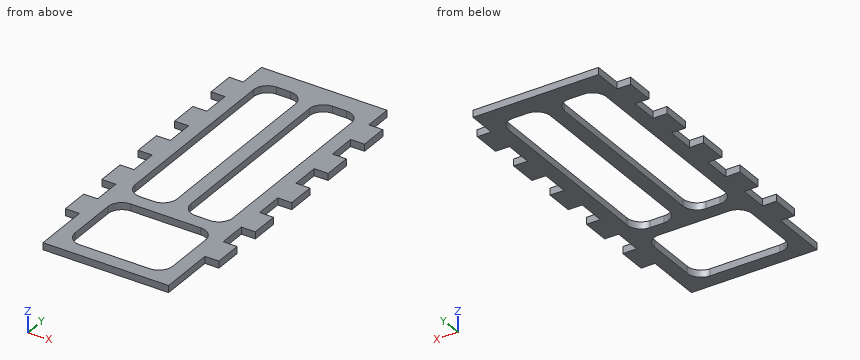
from build123d import *

# Parameters (mm, degrees)
SKETCH1_W           = 57.15
SKETCH1_H           = 152.4
BOSS_EXTRUDE1_DEPTH = 3.175
SKETCH2_W           = 6.35
SKETCH2_H           = 12.7
BOSS_EXTRUDE2_DEPTH = 3.175
LPATTERN1_COUNT     = 5
LPATTERN1_PITCH     = 25.4
SKETCH3_W           = 44.45
SKETCH3_H           = 35.56
CUT_EXTRUDE1_DEPTH  = 3.175
SKETCH4_W           = 19.05
SKETCH4_H           = 95.25
CUT_EXTRUDE2_DEPTH  = 3.175
FILLET1_R           = 6.35


with BuildPart() as part:
    # Sketch1 → Boss-Extrude1 (new body)
    with BuildSketch(Plane.XY):
        with Locations((28.575, 76.2)):
            Rectangle(SKETCH1_W, SKETCH1_H)
    extrude(amount=BOSS_EXTRUDE1_DEPTH)

    # Sketch2 → Boss-Extrude2 (add)
    with BuildSketch(Plane.XY.offset(3.175)):
        with Locations((-3.175, 133.35)):
            Rectangle(SKETCH2_W, SKETCH2_H)
        with Locations((60.325, 133.35)):
            Rectangle(SKETCH2_W, SKETCH2_H)
    boss_extrude2 = extrude(amount=-BOSS_EXTRUDE2_DEPTH)

    # LPattern1: Boss-Extrude2 ×5
    with Locations(*[(0, -i * LPATTERN1_PITCH, 0) for i in range(1, LPATTERN1_COUNT)]):
        add(boss_extrude2)

    # Sketch3 → Cut-Extrude1 (cut)
    with BuildSketch(Plane.XY.offset(3.175)):
        with Locations((28.575, 24.13)):
            Rectangle(SKETCH3_W, SKETCH3_H)
    extrude(amount=-CUT_EXTRUDE1_DEPTH, mode=Mode.SUBTRACT)

    # Sketch4 → Cut-Extrude2 (cut)
    with BuildSketch(Plane.XY.offset(3.175)):
        with Locations((15.875, 95.885)):
            Rectangle(SKETCH4_W, SKETCH4_H)
        with Locations((41.275, 95.885)):
            Rectangle(SKETCH4_W, SKETCH4_H)
    extrude(amount=-CUT_EXTRUDE2_DEPTH, mode=Mode.SUBTRACT)

    # Fillet1
    fillet1_edges = [part.edges().sort_by_distance(p)[0] for p in [
        (6.35, 6.35, 1.5875),
        (6.35, 41.91, 1.5875),
        (50.8, 41.91, 1.5875),
        (50.8, 6.35, 1.5875),
        (6.35, 48.26, 1.5875),
        (6.35, 143.51, 1.5875),
        (25.4, 143.51, 1.5875),
        (25.4, 48.26, 1.5875),
        (31.75, 48.26, 1.5875),
        (31.75, 143.51, 1.5875),
        (50.8, 143.51, 1.5875),
        (50.8, 48.26, 1.5875),
    ]]
    fillet(fillet1_edges, radius=FILLET1_R)


solid = part.part
Can you work these out from the model? Positions are in its coordinate system, mm. Give positions to 0.01 mm unless a question says otherwise; leave off trailing zeros. Order: outer loops, then holes, each group sorted by start corner. A loop starts at its lowest first (then second) coordinate and runs counter-clockwise, first axis right, second up. Notation, with made-up numbers: M 86.25,59 L 99.25,59 A20 cw 99.25,70 Z; hole C -0.75,3 d4. An arc over 180 degrees is marked long. Use one line per item in the form item = value.
Item 1: Will these pins go through, and if not, where does the flat tip stop? pin 1 Ø1 at (y, z) = (24, 2) entering from -X; pin 2 Ø1.6 at (x, z) = (60.5, 1) entering from -Y; pin 3 Ø1.6 at (y, z) = (120.5, 1.5) entering from +X.
Values follow:
pin_1 = 0
pin_2 = 25.4
pin_3 = 57.15
Item 2: If we section it at A-A, the plane y = 124: Write out the boundary of the cut face in (x, z) (3 decimals).
Values follow:
outline = M 0,0 L 6.35,0 L 6.35,3.175 L 0,3.175 Z; M 25.4,0 L 31.75,0 L 31.75,3.175 L 25.4,3.175 Z; M 50.8,0 L 57.15,0 L 57.15,3.175 L 50.8,3.175 Z
Item 3: If we section it at C-C, the plane x = 21: Write out the boundary of the cut face in (y, z) (3 decimals).
Values follow:
outline = M 0,0 L 6.35,0 L 6.35,3.175 L 0,3.175 Z; M 41.91,0 L 48.567,0 L 48.567,3.175 L 41.91,3.175 Z; M 143.203,0 L 152.4,0 L 152.4,3.175 L 143.203,3.175 Z
Item 4: If we section it at D-D, the plane y = 40: Write out the boundary of the cut face in (x, z) (3 decimals).
Values follow:
outline = M 0,0 L 8.16,0 L 8.16,3.175 L 0,3.175 Z; M 48.99,0 L 57.15,0 L 57.15,3.175 L 48.99,3.175 Z
Item 5: If I drill on line 1 along X through (y, z) = (65.5, 2.5); line 2 along X through (y, z) = (108, 2.05); line 3 along Y through (x, z) = (29, 2.15), over which ranges is the centre line in solid material (lowest first)? Write a range as [from, to].
Values follow:
line_1 = [0, 6.35], [25.4, 31.75], [50.8, 57.15]
line_2 = [-6.35, 6.35], [25.4, 31.75], [50.8, 63.5]
line_3 = [0, 6.35], [41.91, 152.4]
Item 6: If we section it at B-B, the plane x = 58.5: Write out the boundary of the cut face in (y, z) (3 decimals), and give its area (3 significant figures).
Values follow:
outline = M 25.4,0 L 38.1,0 L 38.1,3.175 L 25.4,3.175 Z; M 50.8,0 L 63.5,0 L 63.5,3.175 L 50.8,3.175 Z; M 76.2,0 L 88.9,0 L 88.9,3.175 L 76.2,3.175 Z; M 101.6,0 L 114.3,0 L 114.3,3.175 L 101.6,3.175 Z; M 127,0 L 139.7,0 L 139.7,3.175 L 127,3.175 Z
area = 202 mm^2
